from build123d import *

# Parameters (mm, degrees)
SKETCH1_R           = 3.95
BOSS_EXTRUDE1_DEPTH = 6
SKETCH2_W           = 1
SKETCH2_H           = 20
CUT_EXTRUDE1_DEPTH  = 19.493242009
FILLET1_R           = 3
SKETCH3_R           = 1.75
CUT_EXTRUDE2_DEPTH  = 21.426698216
FILLET2_R           = 1


with BuildPart() as part:
    # Sketch1 → Boss-Extrude1 (new body)
    # profile 1 of 3: a face of its own
    with BuildSketch(Plane(origin=(0, 0, 0), x_dir=(1, 0, 0), z_dir=(0, 1, 0))):
        with BuildLine():
            ThreePointArc((9, 0), (-4.974937186, 7.5), (-3.5, -8.291561976))
            Line((-3.5, -8.291561976), (-3.5, -4))
            Line((-3.5, -4), (3.5, -4))
            Line((3.5, -4), (3.5, -8.291561976))
            ThreePointArc((3.5, -8.291561976), (7.5, -4.974937186), (9, 0))
        make_face()
        with Locations(Location((0, 0, 0), (0, 0, 270))):
            Circle(SKETCH1_R, mode=Mode.SUBTRACT)
    # profile 2 of 3: a face of its own
    with BuildSketch(Plane(origin=(0, 0, 0), x_dir=(1, 0, 0), z_dir=(0, 1, 0))):
        with BuildLine():
            Line((-3.5, -4), (-3.5, -8.291561976))
            ThreePointArc((-3.5, -8.291561976), (0, -9), (3.5, -8.291561976))
            Line((3.5, -8.291561976), (3.5, -4))
            Line((3.5, -4), (-3.5, -4))
        make_face()
    # profile 3 of 3: a face of its own
    with BuildSketch(Plane(origin=(0, 0, 0), x_dir=(1, 0, 0), z_dir=(0, 1, 0))):
        with BuildLine():
            Line((-3.5, -8.291561976), (-3.5, -15))
            Line((-3.5, -15), (3.5, -15))
            Line((3.5, -15), (3.5, -8.291561976))
            ThreePointArc((3.5, -8.291561976), (0, -9), (-3.5, -8.291561976))
        make_face()
    extrude(amount=BOSS_EXTRUDE1_DEPTH)

    # Sketch2 → Cut-Extrude1 (cut, through all)
    with BuildSketch(Plane(origin=(0, 6, 0), x_dir=(1, 0, 0), z_dir=(0, 1, 0))):
        with Locations((0, -5)):
            Rectangle(SKETCH2_W, SKETCH2_H)
    extrude(amount=-CUT_EXTRUDE1_DEPTH, mode=Mode.SUBTRACT)

    # Fillet1
    fillet1_edges = [part.edges().sort_by_distance(p)[0] for p in [
        (-2, 0, 15),
        (-2, 6, 15),
        (2, 6, 15),
        (2, 0, 15),
    ]]
    fillet(fillet1_edges, radius=FILLET1_R - 0.0001)  # a hair under: the kernel refuses the full size

    # Sketch3 → Cut-Extrude2 (cut, through all)
    with BuildSketch(Plane(origin=(3.5, 0, 0), x_dir=(0, 0, -1), z_dir=(1, 0, 0))):
        with Locations((-12, 3)):
            Circle(SKETCH3_R)
    extrude(amount=-CUT_EXTRUDE2_DEPTH, mode=Mode.SUBTRACT)

    # Fillet2
    fillet2_edges = [part.edges().sort_by_distance(p)[0] for p in [
        (3.5, 3, 8.291561976),
        (-3.5, 3, 8.291561976),
    ]]
    fillet(fillet2_edges, radius=FILLET2_R)


solid = part.part
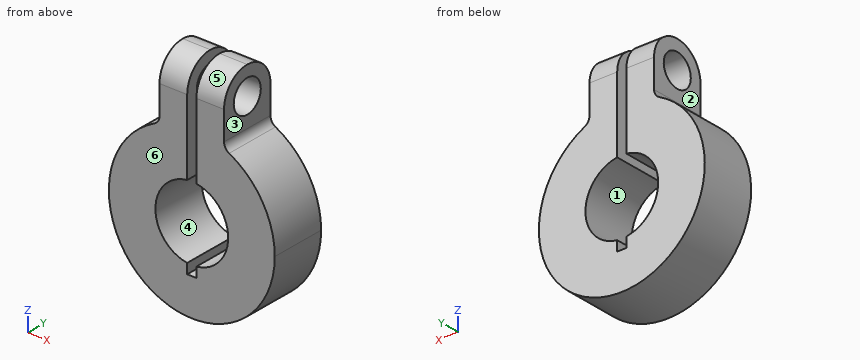
Geometry: final body of the model. Coordinates: model frame, mm. Face numbers are marked on the shaded views. A direction names the side the tool comes from. Round coordinates to 2 decimals unless told otherwise and drop trailing zeros. Loops run counter-clockwise (first coordinate to the right, second up) from the corner with the lowest first, then second, coordinate; pieces in that order, holes last. Notation, with made-up numbers: (43, 78.25) - (75, 78.25) arc R34 ccw to (75, 114.25) - close; hole circle Ø10 at (37.5, 32.5). An arc over 180 degrees is marked (long way). Write each question's results on one line, items separated by ' | '. Start each with the question number.
1) Cut plane A-A on z = 10. Return loops of the section in (x, y), then the cut area to 3 significant figures.
2) Mould query, pull axis Z, two halves, no side actions, for the marked faces 4, 5 and 6. Classes: released by +Z, released by -Z, zero draft, split by the parting line, or undercut.
3) Cut plane C-C on y = 1.5. Return loops of the section in (x, z), then the cut area to 3 significant figures.
4) First-contact query: P1, Ø1.8, axis at y = 2, z = 12.5, coming from the +X side; P2, Ø1.2, axis at y = 4, z = -4.5, coming from the +X side; P3, Ø1.5, axis at x = 7, z = -2.5, coming from the -Y side; P4, Ø1.2, axis at y = 1.5, z = -4.5, coming from the -X side. Flat tips, straight axial feed; report the tip coordinate or a pass-through.
5) Line query: probe 1 along Y at (x, z) = (-2.2, 12); probe 2 along X at (y, z) = (4.6, 13.5); probe 3 along Z at (x, y) = (3.25, 1.5) (3 decimals). Output: solid intervals per line, ascending. Write a range as [from, to].
6) Cut plane B-B on x = -0.75. Count the separate pieces of the cut face and the enclosed holes in it, then the cut area to 3 significant figures.
7) Access query for the marked faces 1, 2 and 3. Directions: +Z, -Z, +X, -X, +Y, -Y. A direction counts if a zero-diameter tool reaches every point of the face in a straight line with its end or side. Return the directions, or none.
Verdict:
1) outline: (-3.5, 0) - (-0.5, 0) - (-0.5, 6) - (-3.5, 6) - close; (0.5, 0) - (3.5, 0) - (3.5, 6) - (0.5, 6) - close | area: 36.0 mm2
2) face 4: undercut | face 5: released by +Z | face 6: zero draft
3) outline: (-4.05, 8.04) arc R9 ccw (long way) to (4.05, 8.04) arc R1 cw to (3.5, 8.93) - (3.5, 11.1) - (0.5, 11.1) - (0.5, 3.92) arc R3.95 cw to (0.5, -3.92) - (0.5, -5) - (-0.5, -5) - (-0.5, -3.92) arc R3.95 cw to (-0.5, 3.92) - (-0.5, 11.1) - (-3.5, 11.1) - (-3.5, 8.93) arc R1 cw to start; (-3.5, 12.9) - (-0.5, 12.9) - (-0.5, 14.6) - (-3.5, 14.6) - close; (0.5, 12.9) - (3.5, 12.9) - (3.5, 14.6) - (0.5, 14.6) - close | area: 224 mm2
4) P1: stops at x = 3.5 | P2: stops at x = 8.11 | P3: stops at y = 0 | P4: stops at x = -8.11
5) probe 1: y = [0, 1.25], [4.75, 6] | probe 2: x = [-3.5, -0.5], [0.5, 3.5] | probe 3: z = [-8.393, -2.245], [2.245, 11.099], [12.901, 14.598]
6) separate pieces: 2 | enclosed holes: 1 | area: 83.8 mm2
7) face 1: +Y, -Y | face 2: +Z, -X, +Y, -Y | face 3: +Z, +X, +Y, -Y
